Model file for the job. Use its own axes, mm. A direction names the side the tool comes from. Coordinates: 2 decimals unless noted, no trailing zeros. Order: outer loops, then holes, each group sorted by start corner. A loop starts at its lowest first (then second) coordinate and runs counter-clockwise, first axis right, second up. Notation, with made-up numbers: M 14,15 L 40,15 A25 ccw 40,44 Z; hole C 50,86.5 d7. An arc over 180 degrees is marked long. Return JSON: item names as keys, results as strings.
```python
from build123d import *

# Parameters (mm, degrees)
BOSS_EXTRUDE1_DEPTH = 160
CUT_EXTRUDE1_DEPTH  = 30


with BuildPart() as part:
    # Sketch1 → Boss-Extrude1 (new body)
    with BuildSketch(Plane(origin=(0, 0, 0), x_dir=(1, 0, 0), z_dir=(0, 1, 0))):
        with BuildLine():
            Line((6.409392014, -3), (6.409392014, 3))
            Line((6.409392014, 3), (9.539392014, 3))
            ThreePointArc((9.539392014, 3), (-10, 0), (9.539392014, -3))
            Line((9.539392014, -3), (6.409392014, -3))
        make_face()
        with BuildLine():
            Line((9.539392014, 3), (6.409392014, 3))
            Line((6.409392014, 3), (6.409392014, -3))
            Line((6.409392014, -3), (9.539392014, -3))
            ThreePointArc((9.539392014, -3), (9.884177258, -1.517576993), (10, 0))
            ThreePointArc((10, 0), (9.884177258, 1.517576993), (9.539392014, 3))
        make_face()
    extrude(amount=BOSS_EXTRUDE1_DEPTH)

    # Sketch1_3 → Cut-Extrude1 (cut)
    with BuildSketch(Plane(origin=(0, 0, 0), x_dir=(1, 0, 0), z_dir=(0, 1, 0))):
        with BuildLine():
            Line((9.539392014, 3), (6.409392014, 3))
            Line((6.409392014, 3), (6.409392014, -3))
            Line((6.409392014, -3), (9.539392014, -3))
            ThreePointArc((9.539392014, -3), (9.884177258, -1.517576993), (10, 0))
            ThreePointArc((10, 0), (9.884177258, 1.517576993), (9.539392014, 3))
        make_face()
    extrude(amount=CUT_EXTRUDE1_DEPTH, mode=Mode.SUBTRACT)


solid = part.part
```
Item 1: Saw through at C-C (z = -7.75). Write the cut outline in (x, y).
Check result:
{"outline": "M -6.32,0 L 6.32,0 L 6.32,160 L -6.32,160 Z"}
Item 2: Wall check: line 1 (Z direction, x = 0.5, y = 99.5); line 2 (X direction, y = 73.5, z = -4.75); line 3 (Z direction, x = 1, y = 67.5). Give the ranges that are in metal, low to high.
Check result:
{"line 1": "z = -9.99 to 9.99", "line 2": "x = -8.8 to 8.8", "line 3": "z = -9.95 to 9.95"}
Item 3: 3-axis set-ups, long thin cutter, end or side, ignore diameter. For faces 1 (the flat face through (0, 160, 0)), 2 (the flat face through (8, 30, 0)): which of +Z, -Z, +X, -X, +Y, -Y reach the whole face in a straight line?
Check result:
{"face 1": "+Z, -Z, +X, -X, +Y", "face 2": "+X, -Y"}
Item 4: Saw through at B-B (x = -7). Write the cut outline in (y, z), and give its area (3 significant figures).
Check result:
{"outline": "M 0,-7.14 L 160,-7.14 L 160,7.14 L 0,7.14 Z", "area": "2,290 mm2"}
Item 5: Drop flat-ended pins along their axis: pin 1 Ø3.5 at (x, y) = (8.5, 17.5) entering from -Z; pin 2 Ø3 at (y, z) = (91, -7) entering from +X; pin 3 Ø1.1 at (x, z) = (8.5, -1) entering from -Y; pin 4 Ø8 at (x, z) = (1, 2) entering from -Y. Give the stop position or say it passes through.
Check result:
{"pin 1": "stops at z = -7.38", "pin 2": "stops at x = 8.35", "pin 3": "stops at y = 30", "pin 4": "stops at y = 0"}
Item 6: Pull direction Z, two halves, no side cores. Call faces 3 (the flat face through (8, 15, -3)), 4 (the flat face through (6.409, 15, 0)), 5 (the flat face through (0, 0, 0)): +Z half, -Z half, draft (parallel to the pull), parting line (faces both ways), or undercut.
Check result:
{"face 3": "undercut", "face 4": "undercut", "face 5": "draft"}
Item 7: Saw through at A-A (y = 135). Write the cut outline in (x, z).
Check result:
{"outline": "C 0,0 d20"}
